Input: dimensioned drawing with shaded views. Units: mm. Origin: part minimum x, y, z. A direction names the side the tool comes from. Give positions to 0.01 mm unless a question says otherwise; leave off trailing zeros. Loops run counter-clockwise (first coordinate to the right, second up) from the corner with the lowest first, then second, coordinate; pieces in that order, holes last. Notation, with made-up numbers: (39.5, -34.5) -> (80.5, -34.5) arc R14 ccw to (80.5, -16.5) -> close; hole circle Ø9 at (11, 26.5). An arc over 180 degrees is marked (long way). One line per question, with ' | ' between items. Start each with the question number.
Item 1: Section C-C on y = 12. Return loops of the section in (x, z).
Item 2: Set-up query: the marked faces 1 and 2. Return all of +Z, -Z, +X, -X, +Y, -Y with unobstructed straight access to the full face (end or side cutting, diameter ignored); none if empty.
Item 3: Material intervals for line 1 along Y through (x, z) = (29.5, 269); line 2 along Z through (x, y) = (51.5, 21); line 3 along Z through (x, y) = (55.5, 49.5), sorted ascending. Write a range as [from, to].
Item 4: Pin query (flat end, axial travel): P1, Ø10, axis at x = 15, y = 6.5, coming from the +Z side; P2, Ø1, axis at x = 34.5, y = 47.5, coming from the +Z side; P3, Ø8, axis at x = 54.5, y = 47.5, coming from the +Z side. Return the tip coordinate at first contact, or that it passes through.
Item 5: Section B-B on y = 27. Return loops of the section in (x, z).
Item 6: Section A-A on x = 40. Return loops of the section in (y, z).
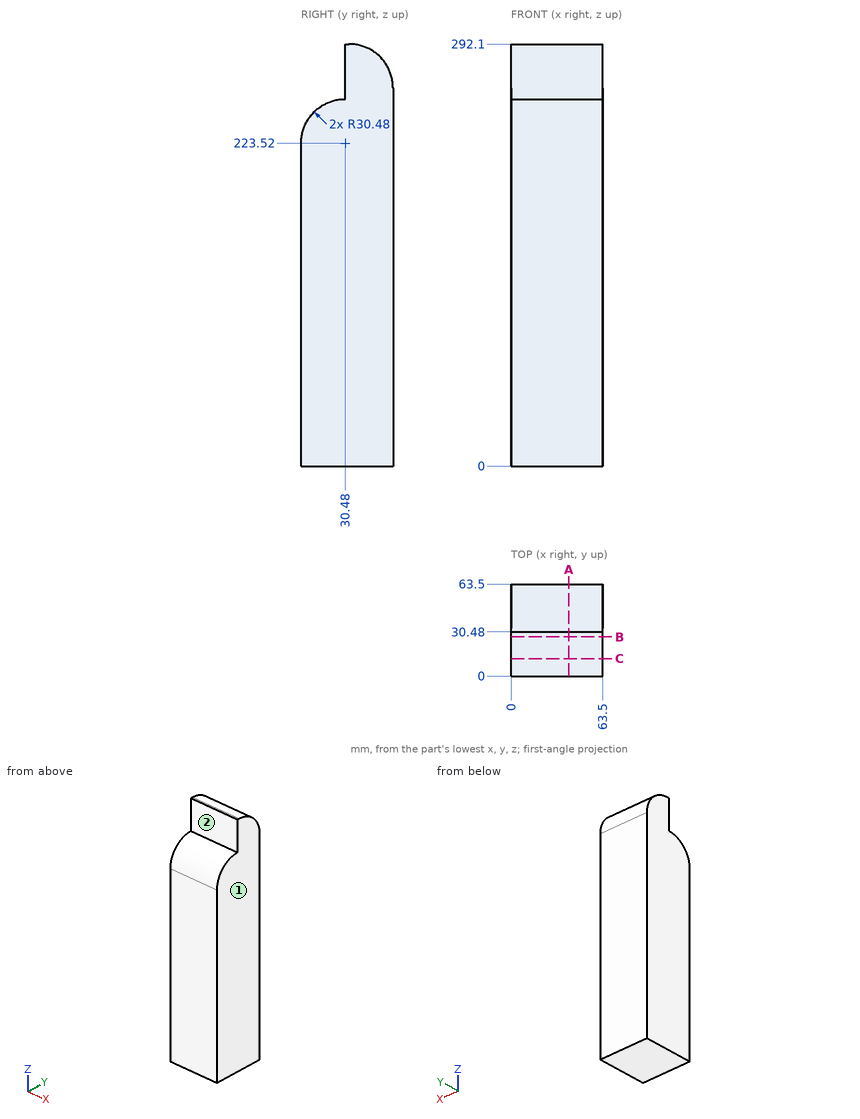
Result sheet:
1) outline: (0, 0) -> (63.5, 0) -> (63.5, 247.76) -> (0, 247.76) -> close
2) face 1: +Z, -Z, +X, +Y, -Y | face 2: +Z, +X, -X, -Y
3) line 1: y = [30.48, 62.59] | line 2: z = [0, 252.49] | line 3: z = [0, 287.26]
4) P1: stops at z = 247.37 | P2: stops at z = 288.7 | P3: stops at z = 290.24
5) outline: (0, 0) -> (63.5, 0) -> (63.5, 253.8) -> (0, 253.8) -> close
6) outline: (0, 0) -> (63.5, 0) -> (63.5, 261.62) arc R30.48 ccw to (33.02, 292.1) -> (30.48, 292.1) -> (30.48, 254) arc R30.48 ccw to (0, 223.52) -> close
